Verification items for the finished model (mm, model axes). Face numbers are marked on the shaded views. A direction names the side the tool comes from. Give positions to 0.01 mm unless a question says otherwise; leave off trailing zeros. Loops run counter-clockwise (first coordinate to the right, second up) from the corner with the lowest first, then second, coordinate; pieces in that order, holes last. Notation, with made-up numbers: (71.5, 20) -> (109.5, 20) arc R23 cw to (109.5, 47) -> close; hole circle Ø7 at (69, 7.25). An arc over 180 degrees is marked (long way). Answer in a Markdown table with one row per item. Add a question column.
Q1. Set-up check for the marked faces 1, 2 and 3: record each of +Z, -Z, +X, -X, +Y, -Y from which the full face is reachable in a straight line by a thin tool's end or side.
Q2. Material ranges on probe 1 along Z at (x, y) = (-8.25, 7); probe 2 along X at (y, z) = (3, 1); probe 3 along X at (y, z) = (6, 4), recorded low to high.
Q3. Gauge pin test, flat ends, axial feed: P1, Ø2, axis at x = 9.5, z = 23, coming from the -Y side; P2, Ø1.3, axis at x = 11, y = 2, coming from the -Z side; P3, Ø4, axis at x = 5.5, y = 3, coming from the +Z side; P4, Ø1, axis at y = 5, z = 7.5, coming from the -X side. Record the tip position at first contact, or that the pin passes through.
Q4. Section check C-C on z = 22.5. Enter the section's corners in (x, y), and give its area (3 significant figures).
Q5. Section check A-A on y = 0.5. Give the number of separate pieces and of enclosed holes in the cut face, and give its area (3 significant figures).
Q6. Section check D-D on x = -4.5. Enter the section's corners in (y, z), and give its area (3 significant figures).
Q7. Release check for a two-part mould opening along Z. For the marked faces 4, 5, 6 and 7 record: pulls with the +Z half, pulls with the -Z half, needs draft (parallel to the pull), parting line crosses it, or undercut.
Q8. Section check B-B on x = 0. Enter the section's corners in (y, z).
```python
from build123d import *

# Parameters (mm, degrees)
BOSS_EXTRUDE1_DEPTH = 53.5
BOSS_EXTRUDE2_DEPTH = 1.5
CUT_EXTRUDE1_DEPTH  = 3
BOSS_EXTRUDE3_DEPTH = 8.5
SKETCH5_R           = 1
CUT_EXTRUDE2_DEPTH  = 10
HOLE1_D             = 2
HOLE1_CBORE_D       = 3.5
HOLE1_CBORE_DEPTH   = 2
CUT_EXTRUDE4_DEPTH  = 3
FILLET1_R           = 2


with BuildPart() as part:
    # Sketch1 → Boss-Extrude1 (new body)
    with BuildSketch(Plane.XY):
        with BuildLine():
            Line((10.25, 0), (10.25, 5))
            ThreePointArc((10.25, 5), (9.224873734, 7.474873734), (6.75, 8.5))
            Line((6.75, 8.5), (-6.75, 8.5))
            ThreePointArc((-6.75, 8.5), (-9.224873734, 7.474873734), (-10.25, 5))
            Line((-10.25, 5), (-10.25, 0))
            Line((-10.25, 0), (-11.75, 0))
            Line((-11.75, 0), (-11.75, 5))
            ThreePointArc((-11.75, 5), (-10.285533906, 8.535533906), (-6.75, 10))
            Line((-6.75, 10), (6.75, 10))
            ThreePointArc((6.75, 10), (10.285533906, 8.535533906), (11.75, 5))
            Line((11.75, 5), (11.75, 0))
            Line((11.75, 0), (10.25, 0))
        make_face()
    extrude(amount=BOSS_EXTRUDE1_DEPTH)

    # Sketch2 → Boss-Extrude2 (add)
    with BuildSketch(Plane.XY):
        with BuildLine():
            Line((-11.75, 0), (11.75, 0))
            Line((11.75, 0), (11.75, 5))
            ThreePointArc((11.75, 5), (10.285533906, 8.535533906), (6.75, 10))
            Line((6.75, 10), (-6.75, 10))
            ThreePointArc((-6.75, 10), (-10.285533906, 8.535533906), (-11.75, 5))
            Line((-11.75, 5), (-11.75, 0))
        make_face()
    extrude(amount=-BOSS_EXTRUDE2_DEPTH)

    # Sketch3 → Cut-Extrude1 (cut)
    with BuildSketch(Plane(origin=(11.75, 0, 0), x_dir=(0, 0, -1), z_dir=(1, 0, 0))):
        with BuildLine():
            Line((-8, 0), (-1.5, 0))
            Line((-1.5, 0), (-1.5, 6))
            ThreePointArc((-1.5, 6), (-2.085786438, 7.414213562), (-3.5, 8))
            Line((-3.5, 8), (-35.5, 8))
            ThreePointArc((-35.5, 8), (-36.914213562, 7.414213562), (-37.5, 6))
            Line((-37.5, 6), (-37.5, 0))
            Line((-37.5, 0), (-8, 0))
        make_face()
    extrude(amount=-CUT_EXTRUDE1_DEPTH, mode=Mode.SUBTRACT)

    # Sketch4 → Boss-Extrude3 (add)
    with BuildSketch(Plane.XZ):
        with BuildLine():
            Line((2.5, 0), (2.5, 4))
            ThreePointArc((2.5, 4), (0, 6.5), (-2.5, 4))
            Line((-2.5, 4), (-2.5, 0))
            Line((-2.5, 0), (2.5, 0))
        make_face()
        with BuildLine():
            Line((10.25, 51.5), (8.25, 51.5))
            ThreePointArc((8.25, 51.5), (5.75, 49), (8.25, 46.5))
            Line((8.25, 46.5), (10.25, 46.5))
            Line((10.25, 46.5), (10.25, 51.5))
        make_face()
        with BuildLine():
            Line((-10.25, 51.5), (-10.25, 46.5))
            Line((-10.25, 46.5), (-8.25, 46.5))
            ThreePointArc((-8.25, 46.5), (-5.75, 49), (-8.25, 51.5))
            Line((-8.25, 51.5), (-10.25, 51.5))
        make_face()
    extrude(amount=-BOSS_EXTRUDE3_DEPTH)

    # Sketch5 → Cut-Extrude2 (cut)
    with BuildSketch(Plane.XZ):
        with Locations((0, 4)):
            Circle(SKETCH5_R)
        with Locations((8.25, 49)):
            Circle(SKETCH5_R)
        with Locations((-8.25, 49)):
            Circle(SKETCH5_R)
    extrude(amount=-CUT_EXTRUDE2_DEPTH, mode=Mode.SUBTRACT)

    # Hole1 (through all)
    with Locations(Plane(origin=(0, 10, 0), x_dir=(1, 0, 0), z_dir=(0, 1, 0))):
        with Locations((0, -4), (-8.25, -49), (8.25, -49)):
            CounterBoreHole(HOLE1_D / 2, HOLE1_CBORE_D / 2, HOLE1_CBORE_DEPTH)

    # Sketch10 → Cut-Extrude4 (cut)
    with BuildSketch(Plane.ZY.offset(11.75)):
        with BuildLine():
            Line((4, 0), (4, 4))
            ThreePointArc((4, 4), (4.585786438, 5.414213562), (6, 6))
            Line((6, 6), (10, 6))
            ThreePointArc((10, 6), (11.414213562, 5.414213562), (12, 4))
            Line((12, 4), (12, 0))
            Line((12, 0), (4, 0))
        make_face()
    extrude(amount=-CUT_EXTRUDE4_DEPTH, mode=Mode.SUBTRACT)

    # Fillet1
    fillet1_edges = [part.edges().sort_by_distance(p)[0] for p in [
        (-11.75, 2.5, -1.5),
        (-10.285533906, 8.535533906, -1.5),
        (0, 10, -1.5),
        (10.285533906, 8.535533906, -1.5),
        (11.75, 2.5, -1.5),
    ]]
    fillet(fillet1_edges, radius=FILLET1_R)


solid = part.part
```
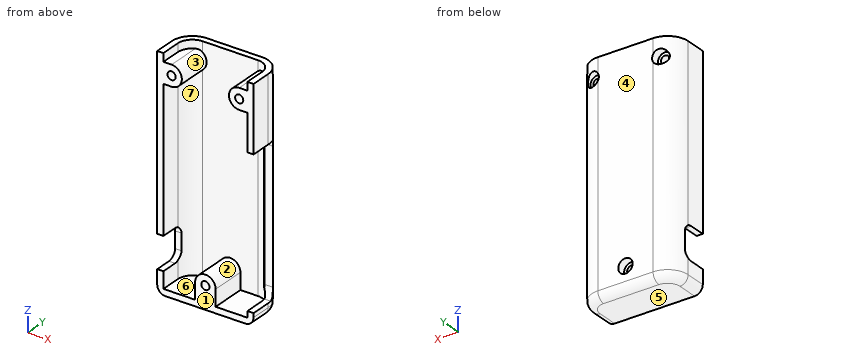
Taken from the geometry:
| question | item | result |
|---|---|---|
| 1 | face 1 | +Z, -Z, +X, -X, -Y |
| 1 | face 2 | +Z, -Y |
| 1 | face 3 | -Y |
| 2 | probe 1 | z = -1.5 to 0, 46.5 to 48, 50 to 51.5 |
| 2 | probe 2 | x = -11.75 to -10.25, -2.5 to 2.5, 10.25 to 11.75 |
| 2 | probe 3 | x = -11.65 to -10.1, -2.5 to -1, 1 to 2.5 |
| 3 | P1 | stops at y = 7.87 |
| 3 | P2 | stops at z = -1.41 |
| 3 | P3 | stops at z = 51.38 |
| 3 | P4 | passes through |
| 4 | outline | (-11.75, 0) -> (-10.25, 0) -> (-10.25, 5) arc R3.5 cw to (-6.75, 8.5) -> (6.75, 8.5) arc R3.5 cw to (8.75, 7.87) -> (8.75, 8) -> (10.75, 8) arc R5 ccw to (6.75, 10) -> (-6.75, 10) arc R5 ccw to (-11.75, 5) -> close |
| 4 | area | 42.8 mm² |
| 5 | separate pieces | 3 |
| 5 | enclosed holes | 3 |
| 5 | area | 188 mm² |
| 6 | outline | (0, -1.5) -> (8, -1.5) arc R2 ccw to (10, 0.5) -> (10, 53.5) -> (8.5, 53.5) -> (8.5, 0) -> (0, 0) -> close |
| 6 | area | 94.4 mm² |
| 7 | face 4 | needs draft |
| 7 | face 5 | pulls with the -Z half |
| 7 | face 6 | undercut |
| 7 | face 7 | undercut |
| 8 | outline | (0, -1.5) -> (8, -1.5) arc R2 ccw to (10, 0.5) -> (10, 2.25) -> (8, 2.25) -> (8, 3) -> (0, 3) -> close; (0, 5) -> (8, 5) -> (8, 5.75) -> (10, 5.75) -> (10, 53.5) -> (8.5, 53.5) -> (8.5, 6.5) -> (0, 6.5) -> close |
